Read the model definition and answer for the solid it produces. Units are mm, in the model's axes. Give positions to 0.01 mm unless a question says otherwise; leave off trailing zeros. Order: outer loops, then holes, each group sorted by start corner. A loop starts at its lowest first (then second) coordinate and runs counter-clockwise, first axis right, second up. Notation, with made-up numbers: M 83.5,9.25 L 114.5,9.25 A26 cw 114.5,35.25 Z; hole C -31,-20 d4. An arc over 180 degrees is marked long. Write item = value, one per line. Start each with the question number.
from build123d import *

# Parameters (mm, degrees)
F1_DEPTH     = 2
F0_W         = 2
F0_H         = 68
F0_W_2       = 103
F0_H_2       = 2
F2_DEPTH     = 2
F3_R         = 2
F4_DEPTH     = 5
F5_R         = 5
F6_T1_DEPTH  = 80
F6_T3_DEPTH  = 115
F6_T6_ANGLE  = 90
F6_T8_ANGLE  = 90
F6_T10_ANGLE = 90
F6_T12_ANGLE = 90


# Not quite as in the source:
# - a fillet or chamfer that OpenCascade refuses, or shapes differently, is made with other operations: its cross-section is extruded or revolved along the edge and cut away or added


with BuildPart() as f1:
    # F0 (on Top) → F1 (new body)
    with BuildSketch(Plane.XY):
        Polygon((-51.5, -43), (51.5, -43), (51.5, -34), (60.5, -34), (60.5, 34), (51.5, 34), (51.5, 43), (-51.5, 43), (-51.5, 34), (-60.5, 34), (-60.5, -34), (-51.5, -34), align=None)
    extrude(amount=F1_DEPTH)

    # F0 (on Top) → F2 (join)
    with BuildSketch(Plane.XY):
        Polygon((-62.5, -45), (-51.5, -45), (-51.5, -43), (-51.5, -34), (-60.5, -34), (-62.5, -34), align=None)
        with Locations((-61.5, 0)):
            Rectangle(F0_W, F0_H)
        with Locations((0, -44)):
            Rectangle(F0_W_2, F0_H_2)
        Polygon((51.5, -45), (62.5, -45), (62.5, -34), (60.5, -34), (51.5, -34), (51.5, -43), align=None)
        with Locations((61.5, 0)):
            Rectangle(F0_W, F0_H)
        Polygon((60.5, 34), (62.5, 34), (62.5, 45), (51.5, 45), (51.5, 43), (51.5, 34), align=None)
        with Locations((0, 44)):
            Rectangle(F0_W_2, F0_H_2)
        Polygon((-62.5, 45), (-62.5, 34), (-60.5, 34), (-51.5, 34), (-51.5, 43), (-51.5, 45), align=None)
    extrude(amount=F2_DEPTH)

    # F3 (on face) → F4 (cut)
    with BuildSketch(Plane.XY.offset(2)):
        with Locations((-57, -39.5)):
            Circle(F3_R)
        with Locations((57, -39.5)):
            Circle(F3_R)
        with Locations((-57, 39.5)):
            Circle(F3_R)
        with Locations((57, 39.5)):
            Circle(F3_R)
    extrude(amount=-F4_DEPTH, mode=Mode.SUBTRACT)

    # F5
    f5_edges = [f1.edges().sort_by_distance(p)[0] for p in [
        (-62.5, 45, 1),
        (62.5, 45, 1),
        (62.5, -45, 1),
        (-62.5, -45, 1),
    ]]
    fillet(f5_edges, radius=F5_R)

    # F6: fillet of radius 5 on 1 edges, made by hand

    # F6_s2 → F6_t1 (cut)
    with BuildSketch(Plane.XZ.offset(-40)):
        with BuildLine():
            ThreePointArc((-62.5, 0), (-60.7360679775, 1.472135955), (-58.5, 2))
            Line((-58.5, 2), (-62.5, 2))
            Line((-62.5, 2), (-62.5, 0))
        make_face()
        with BuildLine():
            ThreePointArc((62.5, 0), (60.7360679775, 1.472135955), (58.5, 2))
            Line((58.5, 2), (62.5, 2))
            Line((62.5, 2), (62.5, 0))
        make_face()
    extrude(amount=F6_T1_DEPTH, mode=Mode.SUBTRACT)

    # F6_s4 → F6_t3 (cut)
    with BuildSketch(Plane.YZ.offset(-57.5)):
        with BuildLine():
            ThreePointArc((-45, 0), (-43.2360679775, 1.472135955), (-41, 2))
            Line((-41, 2), (-45, 2))
            Line((-45, 2), (-45, 0))
        make_face()
        with BuildLine():
            ThreePointArc((45, 0), (43.2360679775, 1.472135955), (41, 2))
            Line((41, 2), (45, 2))
            Line((45, 2), (45, 0))
        make_face()
    extrude(amount=F6_T3_DEPTH, mode=Mode.SUBTRACT)

    # F6_s5 → F6_t6 (revolve, cut)
    with BuildSketch(Plane.XZ.offset(-40)):
        with BuildLine():
            ThreePointArc((-62.5, 0), (-60.7360679775, 1.472135955), (-58.5, 2))
            Line((-58.5, 2), (-62.5, 2))
            Line((-62.5, 2), (-62.5, 0))
        make_face()
    revolve(axis=Axis((-57.5, 40, 2), (0, 0, -1)), revolution_arc=F6_T6_ANGLE, mode=Mode.SUBTRACT)

    # F6_s7 → F6_t8 (revolve, cut)
    with BuildSketch(Plane.YZ.offset(-57.5)):
        with BuildLine():
            ThreePointArc((-45, 0), (-43.2360679775, 1.472135955), (-41, 2))
            Line((-41, 2), (-45, 2))
            Line((-45, 2), (-45, 0))
        make_face()
    revolve(axis=Axis((-57.5, -40, 2), (0, 0, -1)), revolution_arc=F6_T8_ANGLE, mode=Mode.SUBTRACT)

    # F6_s9 → F6_t10 (revolve, cut)
    with BuildSketch(Plane.YZ.offset(57.5)):
        with BuildLine():
            ThreePointArc((-45, 0), (-43.2360679775, 1.472135955), (-41, 2))
            Line((-41, 2), (-45, 2))
            Line((-45, 2), (-45, 0))
        make_face()
    revolve(axis=Axis((57.5, -40, 2), (0, 0, 1)), revolution_arc=F6_T10_ANGLE, mode=Mode.SUBTRACT)

    # F6_s11 → F6_t12 (revolve, cut)
    with BuildSketch(Plane.XZ.offset(-40)):
        with BuildLine():
            ThreePointArc((62.5, 0), (60.7360679775, 1.472135955), (58.5, 2))
            Line((58.5, 2), (62.5, 2))
            Line((62.5, 2), (62.5, 0))
        make_face()
    revolve(axis=Axis((57.5, 40, 2), (0, 0, 1)), revolution_arc=F6_T12_ANGLE, mode=Mode.SUBTRACT)


solid = f1.part
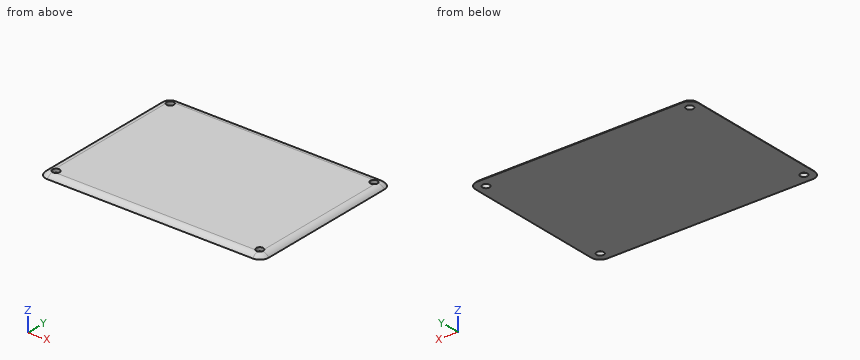
1) Each of these flat-tipped pins is pushed along its axis until it touches: P1, Ø3, axis at x = -57, y = -39.5, coming from the +Z side; P2, Ø5, axis at x = 57, y = 39.5, coming from the -Z side. Where does it stop, or does it pass through?
2) Find section B-B on x = -42. Determine the outline of the cut face in (y, z), plus the area to 3 significant figures.
3) Find section A-A on y = 16. Determine the outline of the cut face in (x, z), plus the area to 3 significant figures.
4) Find the intervals of material crossed by probe 1 along Y at (x, z) = (57, 1.35); probe 2 along Y at (x, z) = (57, 0.45); probe 3 along X at (y, z) = (39.5, 0.55), in increasing order. Write a range as [from, to].
5) Find section C-C on z = 1.2. Count the separate pieces of the cut face and the enclosed holes in it, plus the area to 3 significant figures.
Numbers:
q1.P1 = through
q1.P2 = 0
q2.outline = M -45,0 L 45,0 A5 ccw 41,2 L -41,2 A5 ccw Z
q2.area = 175 mm2
q3.outline = M -62.5,0 L 62.5,0 A5 ccw 58.5,2 L -58.5,2 A5 ccw Z
q3.area = 245 mm2
q4.probe_1 = [-43.47, -41.5], [-37.5, 37.5], [41.5, 43.47]
q4.probe_2 = [-44.62, -41.5], [-37.5, 37.5], [41.5, 44.62]
q4.probe_3 = [-62.02, -59], [-55, 55], [59, 62.02]
q5.separate_pieces = 1
q5.enclosed_holes = 4
q5.area = 10,600 mm2
